Geometry: final body of the model. Coordinates: model frame, mm. Round coordinates to 2 decimals unless told otherwise and drop trailing zeros. Order: outer loops, then holes, each group sorted by start corner. A loop starts at its lowest first (then second) coordinate and runs counter-clockwise, first axis right, second up. Notation, with made-up numbers: (-7.75, 52.25) -> (36.25, 52.25) arc R25 cw to (36.25, 79.25) -> close; hole circle Ø5 at (16, 15.25). An arc over 180 degrees is marked (long way). Put each result on its own line as item: value.
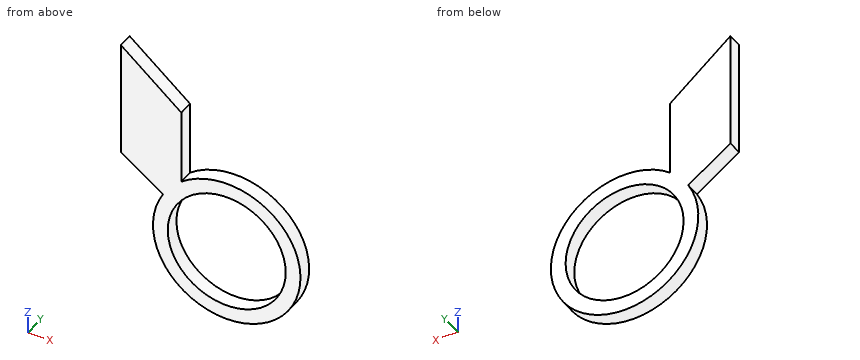
```python
from build123d import *

# Parameters (mm, degrees)
F0_R     = 4
F1_DEPTH = 1


with BuildPart() as f1:
    # F0 (on Front) → F1 (new body)
    with BuildSketch(Plane.XZ):
        with BuildLine():
            Line((-7.178572, 4.5), (-4.31285, 2.529689))
            ThreePointArc((-4.31285, 2.529689), (3.761974, -3.293563), (-3.077627, 3.940585))
            Line((-3.077627, 3.940585), (-3.077627, 9.035675))
            Line((-3.077627, 9.035675), (-7.178572, 12.428572))
            Line((-7.178572, 12.428572), (-7.178572, 4.5))
        make_face()
        Circle(F0_R, mode=Mode.SUBTRACT)
    extrude(amount=F1_DEPTH)


solid = f1.part
```
1. Material intervals for probe 1 along Z at (x, y) = (0, -0.5); probe 2 along X at (y, z) = (-0.2, -3.25); probe 3 along X at (y, z) = (-0.6, 8.5), sorted ascending.
Ans:
probe 1: -5 to -4, 4 to 5
probe 2: -3.8 to -2.33, 2.33 to 3.8
probe 3: -7.18 to -3.08
2. Cut plane B-B on y = -0.75. Return loops of the section in (x, z), and give its area (3 significant figures).
Ans:
outline: (-7.18, 4.5) -> (-4.31, 2.53) arc R5 ccw (long way) to (-3.08, 3.94) -> (-3.08, 9.04) -> (-7.18, 12.43) -> close; hole circle Ø8 at (0, 0)
area: 58.1 mm²
3. Cut plane D-D on z = 5.5. Return loops of the section in (x, y), and give its area (3 significant figures).
Ans:
outline: (-7.18, -1) -> (-3.08, -1) -> (-3.08, 0) -> (-7.18, 0) -> close
area: 4.10 mm²
4. Cut plane A-A on x = 0. Return loops of the section in (y, z), and give its area (3 significant figures).
Ans:
outline: (-1, -5) -> (0, -5) -> (0, -4) -> (-1, -4) -> close; (-1, 4) -> (0, 4) -> (0, 5) -> (-1, 5) -> close
area: 2.00 mm²
5. Cut plane C-C on z = 0. Return loops of the section in (x, y).
Ans:
outline: (-5, -1) -> (-4, -1) -> (-4, 0) -> (-5, 0) -> close; (4, -1) -> (5, -1) -> (5, 0) -> (4, 0) -> close
